Check sheet for the drawn part. Datum: minimum x, y, z corner. Units: mm. A direction names the side the tool comes from. Coordinates: 2 decimals unless noted, no trailing zeros. Loops run counter-clockwise (first coordinate to the right, second up) from the corner with the lowest first, then second, coordinate; pieces in that order, holes last.
Q1. Sectioned sample at D-D (y = 22.5). Enter the section's corners in (x, z), then the cut area to 3 significant figures.
Q2. Material ranges on probe 1 along Y at (x, z) = (1.55, 10); probe 2 along Y at (x, z) = (2.15, 16.5); probe 3 along Y at (x, z) = (1.7, 4.25), recorded low to high.
Q3. Mould release check, pull along Y, two halves, no side actions. Record for the marked faces 1, 2 and 3: +Y half, -Y half, draft (parallel to the pull), parting line (faces both ways), or undercut.
Q4. Go/stop test with a flat-tipped pin: P1, Ø0.9, axis at x = 2, z = 5, coming from the -Y side. Record where the tip stops, or that it passes through.
Q5. Sectioned sample at C-C (z = 16). Enter the section's corners in (x, y), then the cut area to 3 significant figures.
Q6. Sectioned sample at A-A (x = 2.25). Enter the section's corners in (y, z).
Q7. Sectioned sample at B-B (z = 3.25). Enter the section's corners in (x, y).
Q8. Access from +Z, -Z, +X, -X, +Y, -Y to the whole of each face (thin tool, end or side, straight path). Record for the marked faces 4 and 5.
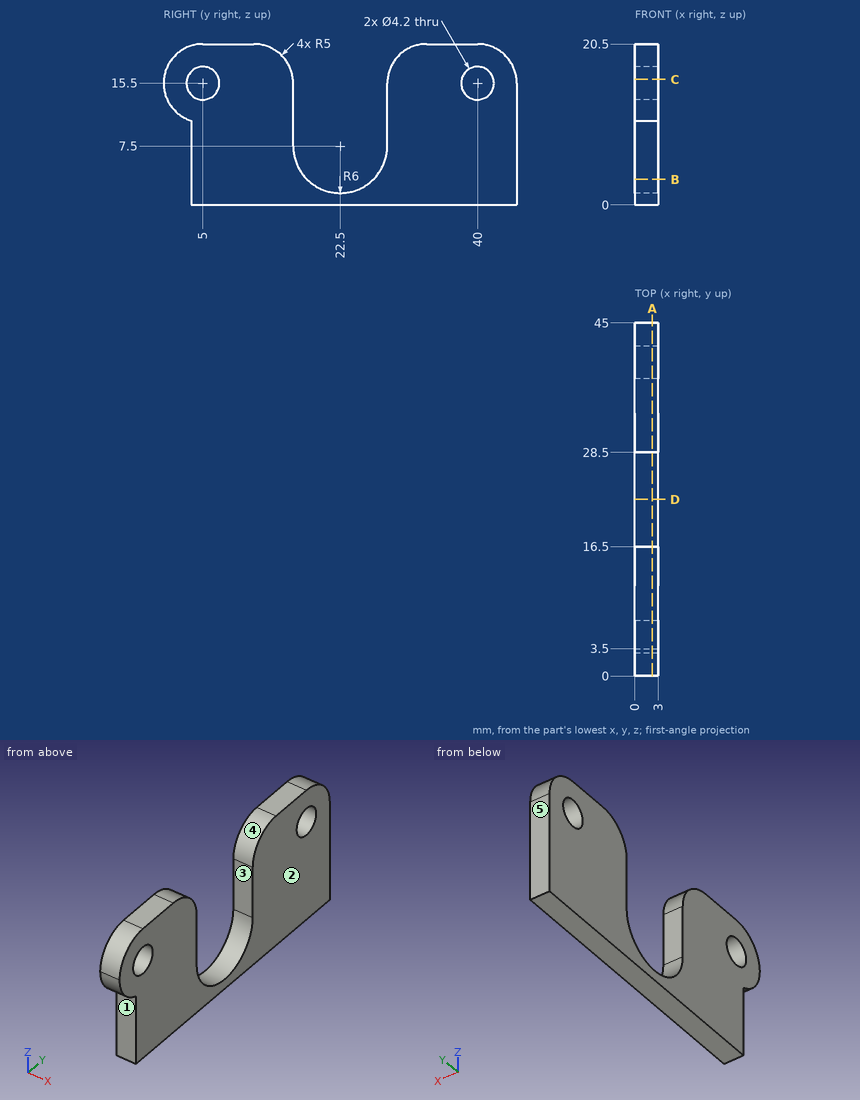
Geometry check:
1. outline: (0, 0) - (3, 0) - (3, 1.5) - (0, 1.5) - close
1. area: 4.50 mm2
2. probe 1: y = 3.5 to 16.5, 28.5 to 45
2. probe 2: y = 0.1 to 3.15, 6.85 to 16.4, 28.6 to 38.15, 41.85 to 44.9
2. probe 3: y = 3.5 to 17.46, 27.54 to 45
3. face 1: -Y half
3. face 2: draft
3. face 3: undercut
4. P1: stops at y = 3.5
5. outline: (0, 0.03) - (3, 0.03) - (3, 2.96) - (0, 2.96) - close; (0, 7.04) - (3, 7.04) - (3, 16.47) - (0, 16.47) - close; (0, 28.53) - (3, 28.53) - (3, 37.96) - (0, 37.96) - close; (0, 42.04) - (3, 42.04) - (3, 44.97) - (0, 44.97) - close
5. area: 74.2 mm2
6. outline: (3.5, 0) - (45, 0) - (45, 15.5) arc R5 ccw to (40, 20.5) - (33.5, 20.5) arc R5 ccw to (28.5, 15.5) - (28.5, 7.5) arc R6 cw to (16.5, 7.5) - (16.5, 15.5) arc R5 ccw to (11.5, 20.5) - (5, 20.5) arc R5 ccw to (3.5, 10.73) - close; hole circle Ø4.2 at (5, 15.5); hole circle Ø4.2 at (40, 15.5)
7. outline: (0, 3.5) - (3, 3.5) - (3, 18.26) - (0, 18.26) - close; (0, 26.74) - (3, 26.74) - (3, 45) - (0, 45) - close
8. face 4: +Z, +X, -X
8. face 5: +Z, -Z, +X, -X, +Y
